```python
from build123d import *

# Parameters (mm, degrees)
BOSS_EXTRUDE1_DEPTH     = 10
CUT_EXTRUDE2_DEPTH      = 10
CUT_EXTRUDE2_DEPTH_BACK = 10


with BuildPart() as part:
    # Sketch1 → Boss-Extrude1 (new body)
    with BuildSketch(Plane(origin=(0, 0, 0), x_dir=(1, 0, 0), z_dir=(0, 1, 0))):
        with BuildLine():
            Line((2, 0), (3.464101615, 0))
            Line((3.464101615, 0), (3.464101615, 2))
            Line((3.464101615, 2), (0, 4))
            Line((0, 4), (-3.464101615, 2))
            Line((-3.464101615, 2), (-3.464101615, -2))
            Line((-3.464101615, -2), (0, -4))
            Line((0, -4), (0, -2))
            ThreePointArc((0, -2), (-1.414213562, 1.414213562), (2, 0))
        make_face()
    extrude(amount=BOSS_EXTRUDE1_DEPTH)

    # Sketch3 → Cut-Extrude2 (cut, two sides)
    with BuildSketch(Plane(origin=(0, 0, 0), x_dir=(0, 0, -1), z_dir=(1, 0, 0))) as cut_extrude2_sk:
        Polygon((-4, 2), (4, 10), (-4, 10), align=None)
    extrude(amount=CUT_EXTRUDE2_DEPTH, mode=Mode.SUBTRACT)
    extrude(cut_extrude2_sk.sketch, amount=-CUT_EXTRUDE2_DEPTH_BACK, mode=Mode.SUBTRACT)


solid = part.part
```
Verification items for the finished model (mm, model axes). A direction names the side the tool comes from. Round coordinates to 2 decimals unless told otherwise and drop trailing zeros. Write each loop counter-clockwise with the first axis right and the second up, starting at its lowest first coordinate (ties: lowest second). Pieces come first, ordered by that corner, then holes.
1. Gauge pin test, flat ends, axial feed: P1, Ø1.5, axis at x = 2, z = -3, coming from the +Y side; P2, Ø1, axis at y = 2.5, z = 3.5, coming from the +X side; P3, Ø3, axis at x = 0, z = 0, coming from the -Y side. Record the tip position at first contact, or that the pin passes through.
2. Section check A-A on z = -1.5. Enter the section's corners in (x, y), plus the area to 3 significant figures.
3. Draft check along Z on faces 3 (the flat face through (-1.756, 1.528, 2.986)), 4 (the cylindrical face through (-0.581, 3.055, -1.914)), 5 (the flat face through (1.756, 4.93, -2.986)), 6 (the flat face through (-1, 0, -2)). Enter one of: +Z half, -Z half, draft (parallel to the pull), parting line (faces both ways), or undercut.
4. Section check C-C on z = -0.5. Enter the section's corners in (x, y), plus the area to 3 significant figures.
5. Scan lines: L1, parallel to Y at x = 0.75, z = -2; L2, parallel to Z at x = -0.5, y = 1.75; L3, parallel to X at y = 3.5, z = -1.25. Record each from-to range of solid material in increasing order.
6. Access from +Z, -Z, +X, -X, +Y, -Y to the whole of each face (thin tool, end or side, straight path). Record for faces 1 (the flat face through (-3.464, 3, 0)), 2 (the flat face through (3, 3, 0)).
7. Section check B-B on y = 1.25. Enter the section's corners in (x, z), plus the area to 3 significant figures.
8. Section check D-D on x = 2.5. Enter the section's corners in (y, z), plus the area to 3 significant figures.
Answer:
1. P1: stops at y = 9.25
1. P2: stops at x = 0
1. P3: passes through
2. outline: (-3.46, 0) - (-1.32, 0) - (-1.32, 7.5) - (-3.46, 7.5) - close; (1.32, 0) - (3.46, 0) - (3.46, 7.5) - (1.32, 7.5) - close
2. area: 32.1 mm2
3. face 3: +Z half
3. face 4: undercut
3. face 5: -Z half
3. face 6: draft
4. outline: (-3.46, 0) - (-1.94, 0) - (-1.94, 6.5) - (-3.46, 6.5) - close; (1.94, 0) - (3.46, 0) - (3.46, 6.5) - (1.94, 6.5) - close
4. area: 19.9 mm2
5. L1: y = 0 to 8
5. L2: z = -3.71 to -1.94, 1.94 to 3.71
5. L3: x = -3.46 to -1.56, 1.56 to 3.46
6. face 1: +Z, -Z, -X, +Y, -Y
6. face 2: +Z, +X, +Y, -Y
7. outline: (-3.46, -2) - (0, -4) - (3.46, -2) - (3.46, 0) - (2, 0) arc R2 cw (long way) to (0, 2) - (0, 4) - (-3.46, 2) - close
7. area: 21.8 mm2
8. outline: (0, -2.56) - (8.56, -2.56) - (6, 0) - (0, 0) - close
8. area: 18.6 mm2
